Can you work these out from the model? Positions are in its coordinate system, mm. A direction names the side the tool comes from. Coordinates: 2 decimals unless noted, no trailing zeros. Order: outer loops, then holes, each group sorted by start corner. A loop starts at its lowest first (then second) coordinate and runs counter-clockwise, first axis right, second up. Notation, with made-up numbers: M 64.25,22 L 77.25,22 A21 cw 77.25,27 Z; hole C 83.5,47 d2. An arc over 180 degrees is marked long. Answer as a JSON object with one key per item and string values.
from build123d import *

# Parameters (mm, degrees)
BOSS_EXTRUDE1_DEPTH = 1.5875
SKETCH2_W           = 2.794
SKETCH2_H           = 2
CUT_EXTRUDE1_DEPTH  = 8.142839509


with BuildPart() as part:
    # Sketch1 → Boss-Extrude1 (new body)
    with BuildSketch(Plane.XY):
        with BuildLine():
            Line((-5.706, -2.5), (5.706, -2.5))
            ThreePointArc((5.706, -2.5), (6.267442784, -2.267442784), (6.5, -1.706))
            Line((6.5, -1.706), (6.5, 1.706))
            ThreePointArc((6.5, 1.706), (6.267442784, 2.267442784), (5.706, 2.5))
            Line((5.706, 2.5), (-5.706, 2.5))
            ThreePointArc((-5.706, 2.5), (-6.267442784, 2.267442784), (-6.5, 1.706))
            Line((-6.5, 1.706), (-6.5, -1.706))
            ThreePointArc((-6.5, -1.706), (-6.267442784, -2.267442784), (-5.706, -2.5))
        make_face()
    extrude(amount=BOSS_EXTRUDE1_DEPTH)

    # Sketch2 → Cut-Extrude1 (cut, through all)
    with BuildSketch(Plane.XY.offset(1.5875)):
        Rectangle(SKETCH2_W, SKETCH2_H)
    extrude(amount=-CUT_EXTRUDE1_DEPTH, mode=Mode.SUBTRACT)


solid = part.part
Item 1: Which directions (+Z, -Z, +X, -X, +Y, -Y) give clear straight access to the entire face, cutting with the end or side of a thin tool? Please do faces 1 (the flat face through (-0.09, 1.15, 1.588)), 2 (the flat face through (0, -1, 1)).
Answers follow:
{"face 1": "+Z, +X, -X, +Y, -Y", "face 2": "+Z, -Z"}
Item 2: I want a section at D-D, the plane y = -2.15. Write out the boundary of the cut face in (x, z).
Answers follow:
{"outline": "M -6.36,0 L 6.36,0 L 6.36,1.59 L -6.36,1.59 Z"}
Item 3: Please list where these lines run through material, in increasing order: line 1 (Y direction, x = -1.25, z = 1); line 2 (X direction, y = 0.8, z = 0.45); line 3 (X direction, y = -1.75, z = 0.2).
Answers follow:
{"line 1": "y = -2.5 to -1, 1 to 2.5", "line 2": "x = -6.5 to -1.4, 1.4 to 6.5", "line 3": "x = -6.5 to 6.5"}
Item 4: I want a section at A-A, the plane y = -0.2. Write out the boundary of the cut face in (x, z).
Answers follow:
{"outline": "M -6.5,0 L -1.4,0 L -1.4,1.59 L -6.5,1.59 Z; M 1.4,0 L 6.5,0 L 6.5,1.59 L 1.4,1.59 Z"}
Item 5: I want a section at C-C, the plane x = 0. Write out the boundary of the cut face in (y, z).
Answers follow:
{"outline": "M -2.5,0 L -1,0 L -1,1.59 L -2.5,1.59 Z; M 1,0 L 2.5,0 L 2.5,1.59 L 1,1.59 Z"}
Item 6: If we mould it in two halves opening along Y, with no side actions, what happens to faces 3 (the flat face through (6.5, 0, 1)), 4 (the flat face through (0, 2.5, 1)), 5 (the flat face through (1.397, 0, 1))? For each: pulls with the +Y half, pulls with the -Y half, needs draft (parallel to the pull), parting line crosses it, or undercut.
Answers follow:
{"face 3": "needs draft", "face 4": "pulls with the +Y half", "face 5": "undercut"}
Item 7: I want a section at B-B, the plane z = 1.2. Write out the boundary of the cut face in (x, y), plus the area to 3 significant figures.
Answers follow:
{"outline": "M -6.5,-1.71 A0.79 ccw -5.71,-2.5 L 5.71,-2.5 A0.79 ccw 6.5,-1.71 L 6.5,1.71 A0.79 ccw 5.71,2.5 L -5.71,2.5 A0.79 ccw -6.5,1.71 Z; hole M -1.4,-1 L 1.4,-1 L 1.4,1 L -1.4,1 Z", "area": "58.9 mm^2"}
